from build123d import *


with BuildPart() as part:
    # Sketch1 → Cabeza_cuello_tambor (revolve)
    with BuildSketch(Plane.XY, mode=Mode.PRIVATE) as cabeza_cuello_tambor_sk:
        Polygon((0, 3.5), (9.8, 3.5), (9.8, -3.5), (6.3, -5), (6.3, -15), (10.5, -16), (10.5, -18), (9, -18), (9, -38), (10.5, -38), (10.5, -40), (6.5, -41), (6.5, -50), (0, -50), align=None)
    revolve(cabeza_cuello_tambor_sk.sketch.rotate(Axis((0, -54, 0), (0, 1, 0)), 90), axis=Axis((0, -54, 0), (0, 1, 0)))

    # Sketch2 → Union_diafisis (revolve)
    with BuildSketch(Plane.XY):
        with BuildLine():
            Line((0, -56.5), (0, -43.5))
            ThreePointArc((0, -43.5), (6.5, -50), (0, -56.5))
        make_face()
    revolve(axis=Axis((0, -60.5, 0), (0, 1, 0)))


solid = part.part
For this review, take the finished solid that the model builds, in its own axes (mm). A direction names the side the tool comes from. Give positions to 0.01 mm unless a question says otherwise; leave off trailing zeros. Order: outer loops, then holes, each group sorted by start corner. A loop starts at its lowest first (then second) coordinate and runs counter-clockwise, first axis right, second up. Notation, with made-up numbers: (0.25, 39) -> (15.25, 39) arc R18 cw to (15.25, 55) -> close; hole circle Ø1 at (28.25, 71.25). An arc over 180 degrees is marked (long way). Write item = value, one per line.
1) We need section A-A, the plane x = 0. Give the boundary of the cut face in (y, z), and give its area (3 significant figures).
Findings:
outline = (-50, -6.5) -> (-41, -6.5) -> (-40, -10.5) -> (-38, -10.5) -> (-38, -9) -> (-18, -9) -> (-18, -10.5) -> (-16, -10.5) -> (-15, -6.3) -> (-5, -6.3) -> (-3.5, -9.8) -> (3.5, -9.8) -> (3.5, 9.8) -> (-3.5, 9.8) -> (-5, 6.3) -> (-15, 6.3) -> (-16, 10.5) -> (-18, 10.5) -> (-18, 9) -> (-38, 9) -> (-38, 10.5) -> (-40, 10.5) -> (-41, 6.5) -> (-50, 6.5) arc R6.5 ccw to start
area = 949 mm^2
2) For faces 4 (the face through (3.937, -4.927, 5.134)), 5 (the face through (-6.623, -0.049, 7.223)), 6 (the face through (3.955, -45.563, 5.158)), list the 3-axis set-ups (+Z, -Z, +X, -X, +Y, -Y) from which the entire face can be reached by the end or side of a thin tool; tool diameter is ignored.
Findings:
face_4 = none
face_5 = +Y
face_6 = -Y
3) To check wall thickness, follow L1, parallel to Y at x = 7.25, z = 6.25; L2, parallel to Y at x = -8, z = -5; L3, parallel to X at y = -3, z = -0.5. State the ranges of each line that lie inside material, in increasing order. Write a range as from..to.
Findings:
L1 = -40.23..-38, -18..-15.78, -3.6..3.5
L2 = -40.27..-38, -18..-15.75, -3.66..3.5
L3 = -9.79..9.79
4) Insertion check: pin 1 (6 mm diameter, centred on x = -3.5, y = -3.5, fed in from +Z); pin 2 (1.5 mm diameter, centred on x = -3, z = -0.5, fed in from -Y); pin 3 (12 mm diameter, centred on x = 4, y = -2.5, fed in from -Z). Each pin has a flat end and moves straight along its axis. Give the tip position at first contact, or say it passes through.
Findings:
pin_1 = 9.79
pin_2 = -56.08
pin_3 = -9.8
5) We need section B-B, the plane z = 0. Give the boundary of the cut face in (x, y).
Findings:
outline = (-10.5, -40) -> (-6.5, -41) -> (-6.5, -50) arc R6.5 ccw to (6.5, -50) -> (6.5, -41) -> (10.5, -40) -> (10.5, -38) -> (9, -38) -> (9, -18) -> (10.5, -18) -> (10.5, -16) -> (6.3, -15) -> (6.3, -5) -> (9.8, -3.5) -> (9.8, 3.5) -> (-9.8, 3.5) -> (-9.8, -3.5) -> (-6.3, -5) -> (-6.3, -15) -> (-10.5, -16) -> (-10.5, -18) -> (-9, -18) -> (-9, -38) -> (-10.5, -38) -> close
6) We need section C-C, the plane y = -20. Give the boundary of the cut face in (x, z).
Findings:
outline = circle Ø18 at (0, 0)
7) Draft analysis for pull direction Y (two halves, no side actions). For faces 1 (the face through (3.993, -15.063, 5.208)), 2 (the face through (-3.2, -17, -10)), 3 (the face through (-2.01, -40.95, -6.39)), state which applies: pulls with the +Y half, pulls with the -Y half, needs draft (parallel to the pull), parting line crosses it, or undercut.
Findings:
face_1 = undercut
face_2 = needs draft
face_3 = pulls with the -Y half
